```python
from build123d import *

# Parameters (mm, degrees)
PAD_DEPTH       = 3
SKETCH001_R     = 2
SKETCH001_R_2   = 1
POCKET_DEPTH    = 3
POCKET001_DEPTH = 3
SKETCH003_R     = 10
SKETCH003_R_2   = 8
PAD001_DEPTH    = 3
PAD002_DEPTH    = 3
SKETCH005_R     = 2
PAD003_DEPTH    = 10
PAD004_DEPTH    = 3


with BuildPart() as part:
    # Sketch → Pad (new body)
    with BuildSketch(Plane.XY):
        with BuildLine():
            ThreePointArc((42.426407, 28.284271), (42.426407, 42.426407), (28.284271, 42.426407))
            Line((28.284271, 42.426407), (5.303301, 22.98097))
            Line((5.303301, 22.98097), (0, 22.98097))
            Line((0, 22.98097), (0, 0))
            Line((0, 0), (22.98097, 0))
            Line((22.98097, 0), (22.98097, 5.303301))
            Line((22.98097, 5.303301), (42.426407, 28.284271))
        make_face()
    extrude(amount=PAD_DEPTH)

    # Sketch001 → Pocket (cut)
    with BuildSketch(Plane.XY.offset(3)):
        with Locations((35.355339, 35.355339)):
            Circle(SKETCH001_R)
        with Locations((38.53732, 38.53732)):
            Circle(SKETCH001_R_2)
        with Locations((32.173359, 38.53732)):
            Circle(SKETCH001_R_2)
        with Locations((32.173359, 32.173359)):
            Circle(SKETCH001_R_2)
        with Locations((38.53732, 32.173359)):
            Circle(SKETCH001_R_2)
    extrude(amount=-POCKET_DEPTH, mode=Mode.SUBTRACT)

    # Sketch002 → Pocket001 (cut)
    with BuildSketch(Plane.XY.offset(3)):
        Polygon((23.452375, 33.116168), (33.116168, 23.452375), (28.549792, 18.05575), (18.05575, 28.549792), align=None)
        Polygon((8.131728, 20.152543), (20.152543, 8.131728), (22.736312, 11.185273), (11.185273, 22.736312), align=None)
        Polygon((12.712046, 24.028197), (24.028197, 12.712046), (27.257908, 16.528977), (16.528977, 27.257908), align=None)
    extrude(amount=-POCKET001_DEPTH, mode=Mode.SUBTRACT)

    # Sketch003 → Pad001 (new body)
    with BuildSketch(Plane.XY.offset(3)):
        with Locations((35.355339, 35.355339)):
            Circle(SKETCH003_R)
        with Locations((35.355339, 35.355339)):
            Circle(SKETCH003_R_2, mode=Mode.SUBTRACT)
    extrude(amount=PAD001_DEPTH)

    # Sketch004 → Pad002 (new body)
    with BuildSketch(Plane.XY.offset(3)):
        Polygon((36.159165, 20.877531), (33.869006, 22.815358), (31.931179, 20.525199), (34.221338, 18.587372), align=None)
        Polygon((25.320081, 14.238818), (27.61024, 12.300992), (29.548067, 14.59115), (27.257908, 16.528977), align=None)
    extrude(amount=PAD002_DEPTH)

    # Sketch005 → Pad003 (new body)
    with BuildSketch(Plane.XY.offset(3)):
        with Locations((10, 10)):
            Circle(SKETCH005_R)
    extrude(amount=PAD003_DEPTH)

    # Sketch006 → Pad004 (new body)
    with BuildSketch(Plane.XY.offset(3)):
        with BuildLine():
            Line((5.303301, 22.98097), (0, 22.98097))
            Line((0, 22.98097), (0, 20.98097))
            Line((0, 20.98097), (4.474874, 20.98097))
            Line((4.474874, 20.98097), (17.437065, 8.018779))
            ThreePointArc((17.437065, 8.018779), (18.819584, 7.479505), (20.152543, 8.131728))
            Line((5.303301, 22.98097), (20.152543, 8.131728))
        make_face()
        with BuildLine():
            Line((22.98097, 5.303301), (22.98097, 0))
            Line((22.98097, 0), (20.98097, 0))
            Line((20.98097, 0), (17.98097, 0))
            Line((17.98097, 0), (15.98097, 0))
            ThreePointArc((19.48097, 3.5), (17.006097, 2.474874), (15.98097, 0))
            ThreePointArc((19.48097, 3.5), (21.449594, 3.977328), (22.98097, 5.303301))
        make_face()
    extrude(amount=PAD004_DEPTH)


solid = part.part
```
Read the model definition and answer for the solid it produces. Units are mm, in the model's axes. A direction names the side the tool comes from. Coordinates: 2 decimals unless noted, no trailing zeros. Write each loop counter-clockwise with the first axis right and the second up, starting at its lowest first coordinate (ties: lowest second). Pieces come first, ordered by that corner, then holes. Notation, with made-up numbers: (-10, 79) -> (5, 79) arc R5 cw to (5, 87) -> close; hole circle Ø10 at (3.25, 8). An arc over 180 degrees is marked (long way). Write item = value, one per line.
(1) Section C-C on y = 16 is taken. Write down the section's boundary in (x, z).
From the geometry:
outline = (0, 0) -> (12.28, 0) -> (12.28, 6) -> (9.46, 6) -> (9.46, 3) -> (0, 3) -> close; (17.92, 0) -> (20.74, 0) -> (20.74, 3) -> (17.92, 3) -> close; (26.81, 0) -> (32.03, 0) -> (32.03, 3) -> (27.88, 3) -> (27.88, 6) -> (26.81, 6) -> close
(2) Section D-D on z = 7.75 is taken. Write down the section's boundary in (x, y), plus the area to 3 significant figures.
From the geometry:
outline = circle Ø4 at (10, 10)
area = 12.6 mm2
(3) For a pull along Y with two mould halves and no side action, classify faces 6 (the face through (18.8, 7.48, 4.48)), 7 (the face through (10, 10, 13)), 8 (the face through (2, 20.981, 4)) as +Y half, -Y half, draft (parallel to the pull), parting line (faces both ways), or undercut.
From the geometry:
face_6 = undercut
face_7 = draft
face_8 = -Y half
(4) Which of the six approach directions +Z, -Z, +X, -X, +Y, -Y give full straight-line access (tool end or side, diameter ignored) to faces 1 (the face through (35.03, 21.833, 4.479)), 2 (the face through (37, 33.7, 3)), 3 (the face through (26.449, 13.283, 4.479)), 4 (the face through (3, 22.981, 3)), 5 (the face through (21.969, 21.818, 1.521))?
From the geometry:
face_1 = +Z, +X
face_2 = +Z
face_3 = +Z, -Y
face_4 = +Z, -Z, -X, +Y
face_5 = +Z, -Z
(5) Given pin 1 Ø13 at (x, y) = (32, 38) entering from +Z; pin 2 Ø2.5 at (x, y) = (38.54, 38.54) entering from +Z; pin 3 Ø5 at (y, z) = (23, 2) entering from +X, each flat-ended and moving along its own axis, determine where each tip first touches the part or whether it passes through.
From the geometry:
pin_1 = 6
pin_2 = 3
pin_3 = 40.07
(6) Straight lines are drawn through the part: L1, parallel to X at y = 13.5, z = 1; L2, parallel to Y at x = 2, z = 2.5; L3, parallel to Y at x = 8.5, z = 1.5. For each, find the intervals that lie inside material, in ascending order. Write a range as from..to.
From the geometry:
L1 = 0..14.78, 20.42..23.24, 24.69..29.92
L2 = 0..22.98
L3 = 0..19.78, 20.46..25.69
(7) Section A-A on x = 10 is taken. Write down the section's boundary in (y, z), plus the area to 3 significant figures.
From the geometry:
outline = (0, 0) -> (18.28, 0) -> (18.28, 6) -> (15.46, 6) -> (15.46, 3) -> (12, 3) -> (12, 13) -> (8, 13) -> (8, 3) -> (0, 3) -> close; (21.73, 0) -> (26.96, 0) -> (26.96, 3) -> (21.73, 3) -> close
area = 119 mm2
